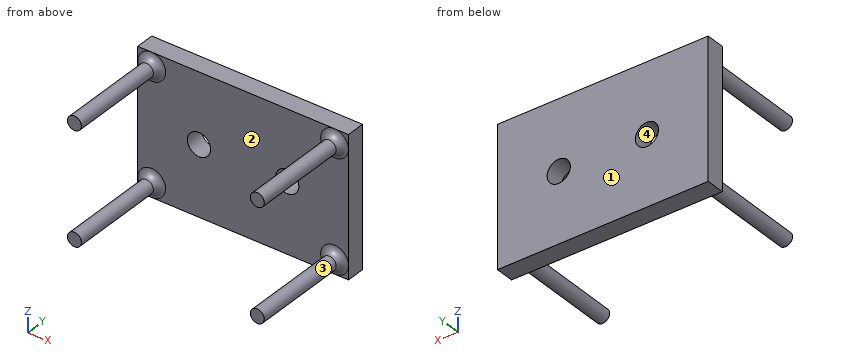
```python
from build123d import *

# Parameters (mm, degrees)
SKETCH1_W           = 45.4
SKETCH1_H           = 30
BOSS_EXTRUDE1_DEPTH = 4
SKETCH2_R           = 2.5
CUT_EXTRUDE1_DEPTH  = 28.500727263
SKETCH3_R           = 1.5
BOSS_EXTRUDE2_DEPTH = 22
FILLET1_R           = 1.5


with BuildPart() as part:
    # Sketch1 → Boss-Extrude1 (new body)
    with BuildSketch(Plane(origin=(0, 0, 0), x_dir=(1, 0, 0), z_dir=(0, 1, 0))):
        Rectangle(SKETCH1_W, SKETCH1_H)
    extrude(amount=BOSS_EXTRUDE1_DEPTH)

    # Sketch2 → Cut-Extrude1 (cut, through all)
    with BuildSketch(Plane(origin=(0, 4, 0), x_dir=(1, 0, 0), z_dir=(0, 1, 0))):
        with Locations(Location((-9.5, 0, 0), (0, 0, 270))):
            Circle(SKETCH2_R)
        with Locations(Location((9.5, 0, 0), (0, 0, 270))):
            Circle(SKETCH2_R)
    extrude(amount=-CUT_EXTRUDE1_DEPTH, mode=Mode.SUBTRACT)

    # Sketch3 → Boss-Extrude2 (add)
    with BuildSketch(Plane.XZ):
        with Locations(Location((-19.7, 12, 0), (0, 0, 270))):
            Circle(SKETCH3_R)
        with Locations(Location((19.7, 12, 0), (0, 0, 270))):
            Circle(SKETCH3_R)
        with Locations(Location((-19.7, -12, 0), (0, 0, 270))):
            Circle(SKETCH3_R)
        with Locations(Location((19.7, -12, 0), (0, 0, 270))):
            Circle(SKETCH3_R)
    extrude(amount=BOSS_EXTRUDE2_DEPTH)

    # Fillet1
    fillet1_edges = [part.edges().sort_by_distance(p)[0] for p in [
        (-19.7, 0, 13.5),
        (19.7, 0, 13.5),
        (-19.7, 0, -10.5),
        (19.7, 0, -10.5),
    ]]
    fillet(fillet1_edges, radius=FILLET1_R - 0.0001)  # a hair under: the kernel refuses the full size


solid = part.part
```
Geometry check sheet. Reference: the model listing, model coordinates, mm. Face numbers are marked on the shaded views. A direction names the side the tool comes from. Coordinates: 2 decimals unless noted, no trailing zeros. Write each loop counter-clockwise with the first axis right and the second up, starting at its lowest first coordinate (ties: lowest second). Pieces come first, ordered by that corner, then holes. Notation, with made-up numbers: M 41,67 L 96,67 A7 cw 96,79 Z; hole C -10,-12 d3. An arc over 180 degrees is marked long. Answer as a JSON object with one key per item and string values.
1. Draft check along X on the marked faces 1 and 2. Enter one of: released by +X, released by -X, zero draft, split by the parting line, or undercut.
Answers below:
{"face 1": "zero draft", "face 2": "undercut"}
2. Section check A-A, the plane x = 9.5. Enter the section's corners in (y, z), plus the area to 3 significant figures.
Answers below:
{"outline": "M 0,-15 L 4,-15 L 4,-2.5 L 0,-2.5 Z; M 0,2.5 L 4,2.5 L 4,15 L 0,15 Z", "area": "100 mm²"}
3. Scan lines: L1, parallel to X at y = 3, z = 0; L2, parallel to Z at x = -18.5, y = -18.5; L3, parallel to Z at x = -9, y = 3. Record each from-to range of solid material in increasing order.
Answers below:
{"L1": "x = -22.7 to -12, -7 to 7, 12 to 22.7", "L2": "z = -12.9 to -11.1, 11.1 to 12.9", "L3": "z = -15 to -2.45, 2.45 to 15"}
4. Go/stop test with flat-tipped pins: pin 1 Ø10 at (x, y) = (16.5, -5.5) entering from +Z; pin 2 Ø12 at (x, y) = (14, -7.5) entering from -Z; pin 3 Ø15 at (x, z) = (0.5, -3.5) entering from -Y. Record where each tip stops, or that it passes through.
Answers below:
{"pin 1": "stops at z = 13.5", "pin 2": "stops at z = -13.5", "pin 3": "stops at y = 0"}
5. Section check B-B, the plane z = 0. Enter the section's corners in (x, y).
Answers below:
{"outline": "M -22.7,0 L -12,0 L -12,4 L -22.7,4 Z; M -7,0 L 7,0 L 7,4 L -7,4 Z; M 12,0 L 22.7,0 L 22.7,4 L 12,4 Z"}
6. Tool access check on the marked faces 3 and 4. Record the directions out of +Z, -Z, +X, -X, +Y, -Y that give a thin tool (end or side, any length) a straight path to the whole face; none if there is none.
Answers below:
{"face 3": "-Y", "face 4": "+Y, -Y"}
